Autodesk Inventor part; units mm, degrees
ref_plane "YZ Plane" through (0, 0, 0) normal (1, 0, 0) x (0, 1, 0)
ref_plane "XZ Plane" through (0, 0, 0) normal (0, 1, 0) x (-1, 0, 0)
ref_plane "XY Plane" through (0, 0, 0) normal (0, 0, 1) x (1, 0, 0)
sketch "Sketch1" plane through (0, 0, 0) normal (0, 0, 1) x (1, 0, 0)
  line L0 (125, -75) -> (-125, -75)
  line L1 (-125, -75) -> (-125, 75)
  line L2 (-125, 75) -> (125, 75)
  line L3 (125, 75) -> (125, -75)
  line L4 (125, -75) -> (-125, 75) construction
  line L5 (-125, -75) -> (125, 75) construction
  point P0 (0, 0)
  dimension "d0" = 250
  dimension "d1" = 150
extrude "Extrusion1" add sketch "Sketch1" along normal blind 5
sketch "Sketch2" plane through (0, 0, 5) normal (0, 0, 1) x (1, 0, 0)
  line L0 (-125, -75) -> (125, -75)
  line L1 (-125, -75) -> (-112, -75)
  line L2 (-112, -75) -> (-112, -57)
  line L3 (-112, -57) -> (-125, -57)
  line L4 (-125, -57) -> (-125, -75)
  line L5 (125, -75) -> (125, 75)
  line L6 (125, -75) -> (112, -75)
  line L7 (112, -75) -> (112, -57)
  line L8 (112, -57) -> (125, -57)
  line L9 (125, -57) -> (125, -75)
  line L10 (125, 75) -> (-125, 75)
  line L11 (-125, 75) -> (-112, 75)
  line L12 (-112, 75) -> (-112, 57)
  line L13 (-112, 57) -> (-125, 57)
  line L14 (-125, 57) -> (-125, 75)
  line L15 (125, 75) -> (112, 75)
  line L16 (112, 75) -> (112, 57)
  line L17 (112, 57) -> (125, 57)
  line L18 (125, 57) -> (125, 75)
  line L19 (-125, 75) -> (-112, 57)
  line L20 (-112, 75) -> (-125, 57)
  line L21 (112, 75) -> (125, 57)
  line L22 (125, 57) -> (125, 75)
  line L23 (112, 57) -> (125, 75)
  line L24 (125, -75) -> (112, -57)
  line L25 (125, -57) -> (112, -75)
  line L26 (-125, -57) -> (-112, -75)
  line L27 (-125, 75) -> (-125, -75)
  line L28 (-112, -57) -> (-125, -75)
  point P0 (0, 0)
  point P1 (-118.5, -66)
  point P2 (-118.5, 66)
  point P3 (118.5, 66)
  point P4 (118.5, -66)
  dimension "d4" = 13
  dimension "d5" = 18
  dimension "d6" = 13
  dimension "d7" = 18
  dimension "d8" = 13
  dimension "d9" = 18
  dimension "d10" = 13
  dimension "d11" = 18
hole "Hole1" at (-118.5, -66, 5) at (118.5, 66, 5) at (118.5, -66, 5) at (-118.5, 66, 5) direction (0, 0, -1) diameter 3.4 end through all counterbore diameter 6.5 counterbore depth 3.4
sketch "Sketch34" plane through (0, 0, 5) normal (0, 0, 1) x (1, 0, 0)
  circle A0 centre (-95, 35) radius 1.7
  line L0 (125, 75) -> (-125, 75)
  line L1 (-125, 75) -> (-125, -75)
  point P0 (0, 0)
  dimension "d166" = 3.4
  dimension "d169" = 40
  dimension "d170" = 30
extrude "ToggleswitchWithCap1" cut sketch "Sketch34" against normal blind 10
sketch "Sketch36" plane through (0, 0, 5) normal (0, 0, 1) x (1, 0, 0)
  circle A0 centre (-65, 35) radius 1.7
  line L0 (125, 75) -> (-125, 75)
  line L1 (-125, 75) -> (-125, -75)
  point P0 (0, 0)
  dimension "d171" = 3.4
  dimension "d172" = 40
  dimension "d173" = 60
extrude "ToggleSwitchWithCap2" cut sketch "Sketch36" against normal through all
sketch "Sketch38" plane through (0, 0, 5) normal (0, 0, 1) x (1, 0, 0)
  line L0 (-71.5, -34.5) -> (-56.5, -34.5)
  line L1 (-56.5, -34.5) -> (-56.5, -55.5)
  line L2 (-56.5, -55.5) -> (-71.5, -55.5)
  line L3 (-71.5, -55.5) -> (-71.5, -34.5)
  line L4 (125, 75) -> (-125, 75)
  line L5 (-125, 75) -> (-125, -75)
  point P0 (0, 0)
  dimension "d181" = 15
  dimension "d182" = 21
  dimension "d185" = 109.5
  dimension "d186" = 53.5
extrude "OnOffToggle" cut sketch "Sketch38" against normal through all
sketch "Sketch17" plane through (0, 0, 5) normal (0, 0, 1) x (1, 0, 0)
  circle A0 centre (-95, -45) radius 9.5
  line L0 (125, 75) -> (-125, 75)
  line L1 (-125, 75) -> (-125, -75)
  point P0 (0, 0)
  point P1 (-104.4472, 75)
  point P2 (-85.5528, 75)
  dimension "d81" = 19
  dimension "d82" = 120
  dimension "d83" = 30
extrude "KeySwitch" cut sketch "Sketch17" against normal through all
sketch "Sketch18" plane through (0, 0, 5) normal (0, 0, 1) x (1, 0, 0)
  circle A0 centre (-5, 50) radius 1.7
  line L0 (-125, 75) -> (-125, -75)
  line L1 (125, 75) -> (-125, 75)
  point P0 (0, 0)
  dimension "d86" = 3.4
  dimension "d98" = 120
  dimension "d99" = 25
extrude "Toggleswitch1" cut sketch "Sketch18" against normal through all
sketch "Sketch19" plane through (0, 0, 5) normal (0, 0, 1) x (1, 0, 0)
  circle A0 centre (25, 50) radius 1.7
  line L0 (125, 75) -> (-125, 75)
  line L1 (-125, 75) -> (-125, -75)
  point P0 (0, 0)
  dimension "d89" = 3.4
  dimension "d100" = 25
  dimension "d101" = 150
extrude "Toggleswitch2" cut sketch "Sketch19" against normal through all
sketch "Sketch20" plane through (0, 0, 5) normal (0, 0, 1) x (1, 0, 0)
  circle A0 centre (55, 50) radius 1.7
  line L0 (125, 75) -> (-125, 75)
  line L1 (-125, 75) -> (-125, -75)
  point P0 (0, 0)
  dimension "d92" = 3.4
  dimension "d102" = 25
  dimension "d103" = 180
extrude "Toggleswitch3" cut sketch "Sketch20" against normal through all
sketch "Sketch21" plane through (0, 0, 5) normal (0, 0, 1) x (1, 0, 0)
  circle A0 centre (85, 50) radius 1.7
  line L0 (125, 75) -> (-125, 75)
  line L1 (-125, 75) -> (-125, -75)
  point P0 (0, 0)
  dimension "d95" = 3.4
  dimension "d104" = 25
  dimension "d105" = 210
extrude "Toggleswitch4" cut sketch "Sketch21" against normal through all
sketch "Sketch22" plane through (0, 0, 5) normal (0, 0, 1) x (1, 0, 0)
  circle A0 centre (-5, 20) radius 6
  line L0 (-125, 75) -> (-125, -75)
  line L1 (125, 75) -> (-125, 75)
  point P0 (0, 0)
  dimension "d106" = 12
  dimension "d109" = 120
  dimension "d110" = 55
extrude "ButtonBlack1" cut sketch "Sketch22" against normal through all
sketch "Sketch23" plane through (0, 0, 5) normal (0, 0, 1) x (1, 0, 0)
  circle A0 centre (25, 20) radius 6
  line L0 (125, 75) -> (-125, 75)
  line L1 (-125, 75) -> (-125, -75)
  point P0 (0, 0)
  dimension "d111" = 12
  dimension "d114" = 55
  dimension "d115" = 150
extrude "ButtonBlack2" cut sketch "Sketch23" against normal through all
sketch "Sketch24" plane through (0, 0, 5) normal (0, 0, 1) x (1, 0, 0)
  circle A0 centre (55, 20) radius 6
  line L0 (125, 75) -> (-125, 75)
  line L1 (-125, 75) -> (-125, -75)
  point P0 (0, 0)
  dimension "d116" = 12
  dimension "d117" = 55
  dimension "d118" = 180
extrude "ButtonBlack3" cut sketch "Sketch24" against normal through all
sketch "Sketch25" plane through (0, 0, 5) normal (0, 0, 1) x (1, 0, 0)
  circle A0 centre (85, 20) radius 6
  line L0 (125, 75) -> (-125, 75)
  line L1 (-125, 75) -> (-125, -75)
  point P0 (0, 0)
  dimension "d121" = 12
  dimension "d122" = 55
  dimension "d123" = 210
extrude "ButtonBlack4" cut sketch "Sketch25" against normal through all
sketch "Sketch26" plane through (0, 0, 5) normal (0, 0, 1) x (1, 0, 0)
  circle A0 centre (-5, -10) radius 6
  line L0 (-125, 75) -> (-125, -75)
  line L1 (125, 75) -> (-125, 75)
  point P0 (0, 0)
  dimension "d126" = 12
  dimension "d127" = 120
  dimension "d128" = 85
extrude "ButtonRed1" cut sketch "Sketch26" against normal through all
sketch "Sketch27" plane through (0, 0, 5) normal (0, 0, 1) x (1, 0, 0)
  circle A0 centre (25, -10) radius 6
  line L0 (125, 75) -> (-125, 75)
  line L1 (-125, 75) -> (-125, -75)
  point P0 (0, 0)
  dimension "d131" = 12
  dimension "d132" = 85
  dimension "d133" = 150
extrude "ButtonRed2" cut sketch "Sketch27" against normal through all
sketch "Sketch28" plane through (0, 0, 5) normal (0, 0, 1) x (1, 0, 0)
  circle A0 centre (55, -10) radius 6
  line L0 (125, 75) -> (-125, 75)
  line L1 (-125, 75) -> (-125, -75)
  point P0 (0, 0)
  dimension "d136" = 12
  dimension "d137" = 85
  dimension "d138" = 180
extrude "ButtonRed3" cut sketch "Sketch28" against normal through all
sketch "Sketch29" plane through (0, 0, 5) normal (0, 0, 1) x (1, 0, 0)
  circle A0 centre (85, -10) radius 6
  line L0 (125, 75) -> (-125, 75)
  line L1 (-125, 75) -> (-125, -75)
  point P0 (0, 0)
  dimension "d141" = 12
  dimension "d142" = 85
  dimension "d143" = 210
extrude "ButtonRed4" cut sketch "Sketch29" against normal through all
sketch "Sketch30" plane through (0, 0, 5) normal (0, 0, 1) x (1, 0, 0)
  circle A0 centre (-5, -45) radius 10
  line L0 (125, 75) -> (-125, 75)
  line L1 (-125, 75) -> (-125, -75)
  point P0 (0, 0)
  dimension "d146" = 20
  dimension "d147" = 120
  dimension "d148" = 120
extrude "RotaryEncoder1" cut sketch "Sketch30" against normal through all
sketch "Sketch31" plane through (0, 0, 5) normal (0, 0, 1) x (1, 0, 0)
  circle A0 centre (25, -45) radius 10
  line L0 (125, 75) -> (-125, 75)
  line L1 (-125, 75) -> (-125, -75)
  point P0 (0, 0)
  dimension "d151" = 20
  dimension "d152" = 120
  dimension "d153" = 150
extrude "RotaryEncoder2" cut sketch "Sketch31" against normal through all
sketch "Sketch32" plane through (0, 0, 5) normal (0, 0, 1) x (1, 0, 0)
  circle A0 centre (55, -45) radius 10
  line L0 (125, 75) -> (-125, 75)
  line L1 (-125, 75) -> (-125, -75)
  point P0 (0, 0)
  dimension "d156" = 20
  dimension "d157" = 120
  dimension "d158" = 180
extrude "RotaryEncoder3" cut sketch "Sketch32" against normal through all
sketch "Sketch33" plane through (0, 0, 5) normal (0, 0, 1) x (1, 0, 0)
  circle A0 centre (85, -45) radius 10
  line L0 (125, 75) -> (-125, 75)
  line L1 (-125, 75) -> (-125, -75)
  point P0 (0, 0)
  dimension "d161" = 20
  dimension "d162" = 120
  dimension "d163" = 210
extrude "RotaryEncoder4" cut sketch "Sketch33" against normal through all
properties part number "Box Top"
Geometry: final body of the model. Coordinates: model frame, mm. A direction names the side the tool comes from. Give positions to 0.01 mm unless a question says otherwise; leave off trailing zeros. Write each loop counter-clockwise with the first axis right and the second up, starting at its lowest first coordinate (ties: lowest second). Pieces come first, ordered by that corner, then holes. Notation, with made-up numbers: (29, -23.5) -> (71, -23.5) arc R19 ccw to (71, -8.5) -> close; hole circle Ø1 at (82, 71). An arc over 180 degrees is marked (long way). Answer as a JSON object with one key per item and string values.
1. Cut plane C-C on y = 20. Output: boundary loops of the cut face in (x, z).
Ans:
{"outline": "(-125, 0) -> (-11, 0) -> (-11, 5) -> (-125, 5) -> close; (1, 0) -> (19, 0) -> (19, 5) -> (1, 5) -> close; (31, 0) -> (49, 0) -> (49, 5) -> (31, 5) -> close; (61, 0) -> (79, 0) -> (79, 5) -> (61, 5) -> close; (91, 0) -> (125, 0) -> (125, 5) -> (91, 5) -> close"}
2. Cut plane B-B on z = 2.7. Count the separate pieces of the cut face and the enclosed holes in it, and give its area (3 significant figures).
Ans:
{"separate pieces": "1", "enclosed holes": "24", "area": "34,600 mm^2"}
3. Ray query, probe 1 along Y at (x, z) = (-118.5, 3.65); probe 2 along Y at (x, z) = (55, 3.6); probe 3 along Y at (x, z) = (-65, 1.4). Return the intervals inside material, ascending. Write a range as from..to.
Ans:
{"probe 1": "y = -75..-69.25, -62.75..62.75, 69.25..75", "probe 2": "y = -75..-55, -35..-16, -4..14, 26..48.3, 51.7..75", "probe 3": "y = -75..-55.5, -34.5..33.3, 36.7..75"}
4. Cut plane A-A on y = -45. Output: boundary loops of the cut face in (x, z).
Ans:
{"outline": "(-125, 0) -> (-104.5, 0) -> (-104.5, 5) -> (-125, 5) -> close; (-85.5, 0) -> (-71.5, 0) -> (-71.5, 5) -> (-85.5, 5) -> close; (-56.5, 0) -> (-15, 0) -> (-15, 5) -> (-56.5, 5) -> close; (5, 0) -> (15, 0) -> (15, 5) -> (5, 5) -> close; (35, 0) -> (45, 0) -> (45, 5) -> (35, 5) -> close; (65, 0) -> (75, 0) -> (75, 5) -> (65, 5) -> close; (95, 0) -> (125, 0) -> (125, 5) -> (95, 5) -> close"}
5. Mould query, pull axis Y, two halves, no side actions, for faces 1 (the flat face through (-2, 1, 0)), 2 (the cylindrical face through (-9.76, 16.35, 2.54)), 3 (the flat face through (-2, 75, 2)). Classes: pulls with the +Y half, pulls with the -Y half, needs draft (parallel to the pull), parting line crosses it, or undercut.
Ans:
{"face 1": "needs draft", "face 2": "undercut", "face 3": "pulls with the +Y half"}
6. Contact query for a flat-ended pin moving along its axis: pin 1 (8.5 mm diameter, centred on x = 118.5, y = -66, fed in from +Z). Output: stop coordinate, or through.
Ans:
{"pin 1": "stops at z = 5"}
7. Access query for faces 4 (the flat face through (-2, 1, 5)), 5 (the cylindrical face through (121.673, -65.295, 3.276)), 6 (the flat face through (-64, -55.5, 3)). Directions: +Z, -Z, +X, -X, +Y, -Y. A direction counts if a zero-diameter tool reaches every point of the face in a straight line with its end or side. Return the directions, or none.
Ans:
{"face 4": "+Z, +X, -X, +Y, -Y", "face 5": "+Z", "face 6": "+Z, -Z"}
